from build123d import *

# Parameters (mm, degrees)
SKETCH1_W           = 270
SKETCH1_H           = 35
BOSS_EXTRUDE1_DEPTH = 10
SKETCH2_W           = 270
SKETCH2_H           = 26
BOSS_EXTRUDE2_DEPTH = 1
CUT_EXTRUDE1_REACH  = 141.821
SKETCH3_R           = 1.75
CUT_EXTRUDE3_REACH  = 141.896
SKETCH4_R           = 8
SKETCH5_R           = 10
CUT_EXTRUDE4_DEPTH  = 1.5
CUT_EXTRUDE5_START  = -1.5
SKETCH6_R           = 10
CUT_EXTRUDE5_DEPTH  = 1.5
CUT_EXTRUDE14_REACH = 141.896
SKETCH20_W          = 17
SKETCH20_H          = 15
BOSS_EXTRUDE5_DEPTH = 11
SKETCH21_R          = 4.25
CUT_EXTRUDE15_DEPTH = 9
FILLET1_R           = 7
CUT_EXTRUDE16_REACH = 146.381
SKETCH22_R          = 1.75
SKETCH24_R          = 3
CUT_EXTRUDE17_DEPTH = 5
BOSS_EXTRUDE6_DEPTH = 11
FILLET2_R           = 20
FILLET3_R           = 30
CHAMFER1_SIZE       = 1


# Some blends are built 0.0001 mm under size
with BuildPart() as part:
    # Sketch1 → Boss-Extrude1 (new body)
    with BuildSketch(Plane.XY):
        with Locations((0, -17.5)):
            Rectangle(SKETCH1_W, SKETCH1_H)
    extrude(amount=BOSS_EXTRUDE1_DEPTH)

    # Sketch2 → Boss-Extrude2 (add)
    with BuildSketch(Plane.XY.offset(10)):
        with Locations((0, -22)):
            Rectangle(SKETCH2_W, SKETCH2_H)
    extrude(amount=BOSS_EXTRUDE2_DEPTH)

    # Sketch3 → Cut-Extrude1 (cut, up to next)
    with BuildSketch(Plane.XY.offset(10), mode=Mode.PRIVATE) as cut_extrude1_sk1:
        with Locations((-130, -4.5)):
            Circle(SKETCH3_R)
    cut_extrude1_tool1 = extrude(cut_extrude1_sk1.sketch, amount=-CUT_EXTRUDE1_REACH, mode=Mode.PRIVATE) & part.part
    # Sketch3 → Cut-Extrude1 (cut, up to next)
    with BuildSketch(Plane.XY.offset(10), mode=Mode.PRIVATE) as cut_extrude1_sk2:
        with Locations((-110, -4.5)):
            Circle(SKETCH3_R)
    cut_extrude1_tool2 = extrude(cut_extrude1_sk2.sketch, amount=-CUT_EXTRUDE1_REACH, mode=Mode.PRIVATE) & part.part
    # Sketch3 → Cut-Extrude1 (cut, up to next)
    with BuildSketch(Plane.XY.offset(10), mode=Mode.PRIVATE) as cut_extrude1_sk3:
        with Locations((-90, -4.5)):
            Circle(SKETCH3_R)
    cut_extrude1_tool3 = extrude(cut_extrude1_sk3.sketch, amount=-CUT_EXTRUDE1_REACH, mode=Mode.PRIVATE) & part.part
    # Sketch3 → Cut-Extrude1 (cut, up to next)
    with BuildSketch(Plane.XY.offset(10), mode=Mode.PRIVATE) as cut_extrude1_sk4:
        with Locations((-70, -4.5)):
            Circle(SKETCH3_R)
    cut_extrude1_tool4 = extrude(cut_extrude1_sk4.sketch, amount=-CUT_EXTRUDE1_REACH, mode=Mode.PRIVATE) & part.part
    # Sketch3 → Cut-Extrude1 (cut, up to next)
    with BuildSketch(Plane.XY.offset(10), mode=Mode.PRIVATE) as cut_extrude1_sk5:
        with Locations((-50, -4.5)):
            Circle(SKETCH3_R)
    cut_extrude1_tool5 = extrude(cut_extrude1_sk5.sketch, amount=-CUT_EXTRUDE1_REACH, mode=Mode.PRIVATE) & part.part
    # Sketch3 → Cut-Extrude1 (cut, up to next)
    with BuildSketch(Plane.XY.offset(10), mode=Mode.PRIVATE) as cut_extrude1_sk6:
        with Locations((-30, -4.5)):
            Circle(SKETCH3_R)
    cut_extrude1_tool6 = extrude(cut_extrude1_sk6.sketch, amount=-CUT_EXTRUDE1_REACH, mode=Mode.PRIVATE) & part.part
    # Sketch3 → Cut-Extrude1 (cut, up to next)
    with BuildSketch(Plane.XY.offset(10), mode=Mode.PRIVATE) as cut_extrude1_sk7:
        with Locations((-10, -4.5)):
            Circle(SKETCH3_R)
    cut_extrude1_tool7 = extrude(cut_extrude1_sk7.sketch, amount=-CUT_EXTRUDE1_REACH, mode=Mode.PRIVATE) & part.part
    # Sketch3 → Cut-Extrude1 (cut, up to next)
    with BuildSketch(Plane.XY.offset(10), mode=Mode.PRIVATE) as cut_extrude1_sk8:
        with Locations((10, -4.5)):
            Circle(SKETCH3_R)
    cut_extrude1_tool8 = extrude(cut_extrude1_sk8.sketch, amount=-CUT_EXTRUDE1_REACH, mode=Mode.PRIVATE) & part.part
    # Sketch3 → Cut-Extrude1 (cut, up to next)
    with BuildSketch(Plane.XY.offset(10), mode=Mode.PRIVATE) as cut_extrude1_sk9:
        with Locations((30, -4.5)):
            Circle(SKETCH3_R)
    cut_extrude1_tool9 = extrude(cut_extrude1_sk9.sketch, amount=-CUT_EXTRUDE1_REACH, mode=Mode.PRIVATE) & part.part
    # Sketch3 → Cut-Extrude1 (cut, up to next)
    with BuildSketch(Plane.XY.offset(10), mode=Mode.PRIVATE) as cut_extrude1_sk10:
        with Locations((50, -4.5)):
            Circle(SKETCH3_R)
    cut_extrude1_tool10 = extrude(cut_extrude1_sk10.sketch, amount=-CUT_EXTRUDE1_REACH, mode=Mode.PRIVATE) & part.part
    # Sketch3 → Cut-Extrude1 (cut, up to next)
    with BuildSketch(Plane.XY.offset(10), mode=Mode.PRIVATE) as cut_extrude1_sk11:
        with Locations((70, -4.5)):
            Circle(SKETCH3_R)
    cut_extrude1_tool11 = extrude(cut_extrude1_sk11.sketch, amount=-CUT_EXTRUDE1_REACH, mode=Mode.PRIVATE) & part.part
    # Sketch3 → Cut-Extrude1 (cut, up to next)
    with BuildSketch(Plane.XY.offset(10), mode=Mode.PRIVATE) as cut_extrude1_sk12:
        with Locations((90, -4.5)):
            Circle(SKETCH3_R)
    cut_extrude1_tool12 = extrude(cut_extrude1_sk12.sketch, amount=-CUT_EXTRUDE1_REACH, mode=Mode.PRIVATE) & part.part
    add(cut_extrude1_tool1.solids().sort_by_distance((-130, -4.5, 10))[0], mode=Mode.SUBTRACT)
    add(cut_extrude1_tool2.solids().sort_by_distance((-110, -4.5, 10))[0], mode=Mode.SUBTRACT)
    add(cut_extrude1_tool3.solids().sort_by_distance((-90, -4.5, 10))[0], mode=Mode.SUBTRACT)
    add(cut_extrude1_tool4.solids().sort_by_distance((-70, -4.5, 10))[0], mode=Mode.SUBTRACT)
    add(cut_extrude1_tool5.solids().sort_by_distance((-50, -4.5, 10))[0], mode=Mode.SUBTRACT)
    add(cut_extrude1_tool6.solids().sort_by_distance((-30, -4.5, 10))[0], mode=Mode.SUBTRACT)
    add(cut_extrude1_tool7.solids().sort_by_distance((-10, -4.5, 10))[0], mode=Mode.SUBTRACT)
    add(cut_extrude1_tool8.solids().sort_by_distance((10, -4.5, 10))[0], mode=Mode.SUBTRACT)
    add(cut_extrude1_tool9.solids().sort_by_distance((30, -4.5, 10))[0], mode=Mode.SUBTRACT)
    add(cut_extrude1_tool10.solids().sort_by_distance((50, -4.5, 10))[0], mode=Mode.SUBTRACT)
    add(cut_extrude1_tool11.solids().sort_by_distance((70, -4.5, 10))[0], mode=Mode.SUBTRACT)
    add(cut_extrude1_tool12.solids().sort_by_distance((90, -4.5, 10))[0], mode=Mode.SUBTRACT)

    # Sketch4 → Cut-Extrude3 (cut, up to next)
    with BuildSketch(Plane.XY.offset(11), mode=Mode.PRIVATE) as cut_extrude3_sk1:
        with Locations((123, -24.5)):
            Circle(SKETCH4_R)
    cut_extrude3_tool1 = extrude(cut_extrude3_sk1.sketch, amount=-CUT_EXTRUDE3_REACH, mode=Mode.PRIVATE) & part.part
    add(cut_extrude3_tool1.solids().sort_by_distance((123, -24.5, 11))[0], mode=Mode.SUBTRACT)

    # Sketch5 → Cut-Extrude4 (cut)
    with BuildSketch(Plane.XY.offset(11)):
        with Locations((123, -24.5)):
            Circle(SKETCH5_R)
    extrude(amount=-CUT_EXTRUDE4_DEPTH, mode=Mode.SUBTRACT)

    # Sketch6 → Cut-Extrude5 (cut)
    with BuildSketch(Plane(origin=(0, 0, 0), x_dir=(-1, 0, 0), z_dir=(0, 0, -1)).offset(CUT_EXTRUDE5_START)):
        with Locations(Location((-123, -24.5, 0), (0, 0, 180))):
            Circle(SKETCH6_R)
    extrude(amount=CUT_EXTRUDE5_DEPTH, mode=Mode.SUBTRACT)

    # Sketch19 → Cut-Extrude14 (cut, up to next)
    with BuildSketch(Plane.XY.offset(11), mode=Mode.PRIVATE) as cut_extrude14_sk1:
        with BuildLine():
            Line((-135, -12), (-135, -35))
            Line((-135, -35), (-126.157637496, -35))
            ThreePointArc((-126.157637496, -35), (-129.258467146, -22.992390109), (-135, -12))
        make_face()
    cut_extrude14_tool1 = extrude(cut_extrude14_sk1.sketch, amount=-CUT_EXTRUDE14_REACH, mode=Mode.PRIVATE) & part.part
    add(cut_extrude14_tool1.solids().sort_by_distance((-131.679264, -26.580863, 11))[0], mode=Mode.SUBTRACT)

    # Sketch20 → Boss-Extrude5 (add)
    with BuildSketch(Plane.XY.offset(11)):
        with Locations((-89.087637496, -42.5)):
            Rectangle(SKETCH20_W, SKETCH20_H)
    extrude(amount=-BOSS_EXTRUDE5_DEPTH)

    # Sketch21 → Cut-Extrude15 (cut)
    with BuildSketch(Plane(origin=(0, 0, 0), x_dir=(-1, 0, 0), z_dir=(0, 0, -1))):
        with Locations((89.087637496, -41)):
            Circle(SKETCH21_R)
    extrude(amount=-CUT_EXTRUDE15_DEPTH, mode=Mode.SUBTRACT)

    # Fillet1
    fillet1_edges = [part.edges().sort_by_distance(p)[0] for p in [
        (-80.587637496, -50, 5.5),
        (-80.587637496, -35, 5.5),
        (-97.587637496, -35, 5.5),
        (-97.587637496, -50, 5.5),
    ]]
    fillet(fillet1_edges, radius=FILLET1_R)

    # Sketch22 → Cut-Extrude16 (cut, up to next)
    with BuildSketch(Plane.XY.offset(11), mode=Mode.PRIVATE) as cut_extrude16_sk1:
        with Locations((-75, -27)):
            Circle(SKETCH22_R)
    cut_extrude16_tool1 = extrude(cut_extrude16_sk1.sketch, amount=-CUT_EXTRUDE16_REACH, mode=Mode.PRIVATE) & part.part
    add(cut_extrude16_tool1.solids().sort_by_distance((-75, -27, 11))[0], mode=Mode.SUBTRACT)

    # Sketch24 → Cut-Extrude17 (cut)
    with BuildSketch(Plane.XY.offset(11)):
        with Locations((-75, -27)):
            Circle(SKETCH24_R)
    extrude(amount=-CUT_EXTRUDE17_DEPTH, mode=Mode.SUBTRACT)

    # Sketch25 → Boss-Extrude6 (add)
    with BuildSketch(Plane.XY.offset(11)):
        with BuildLine():
            Line((109.630258043, -35), (135, -35))
            Line((135, -35), (135, -12.458405421))
            ThreePointArc((135, -12.458405421), (134.291586239, -37.208268183), (109.630258043, -35))
        make_face()
    extrude(amount=-BOSS_EXTRUDE6_DEPTH)

    # Fillet2
    fillet2_edges = [part.edges().sort_by_distance(p)[0] for p in [
        (109.630258043, -35, 5.5),
        (135, -12.458405421, 5.5),
    ]]
    fillet(fillet2_edges, radius=FILLET2_R)

    # Fillet3
    # the kernel refuses this fillet: 30 mm, written as the material it takes off along each edge
    with BuildSketch(Plane(origin=(135, 0, -59.556893558), x_dir=(0.15687721441573954, -0.9876181142512312, 0), z_dir=(0, 0, 1))) as fillet3_piece_1:
        with BuildLine():
            CenterArc((25.891295603, -28.234103195), FILLET3_R, 109.756652653, 61.217662553)
            Line((-3.737247824, -23.527786763), (-6.700102167, -23.057155119))
            Line((-6.700102167, -23.057155119), (-2.962854343, 0.470631643))
            Line((-2.962854343, 0.470631643), (0.470631643, 2.962854343))
            ThreePointArc((0.470631643, 2.962854343), (6.323083142, 2.033227521), (14.736437724, 2.823410319))
            Line((14.736437724, 2.823410319), (15.750515713, 0))
        make_face()
    extrude(amount=129.113787116, mode=Mode.SUBTRACT)

    # Chamfer1
    chamfer1_edges = [part.edges().sort_by_distance(p)[0] for p in [
        (-97.587637496, -42.5, 11),
        (-89.087637496, -50, 11),
        (-80.587637496, -42.5, 11),
        (14.233001219, -35, 11),
        (-82.637890028, -47.949747468, 11),
        (-95.537384964, -47.949747468, 11),
        (-99.637890028, -37.050252532, 11),
        (-78.537384964, -37.050252532, 11),
        (-78, -27, 11),
        (-135, -10.5, 11),
        (134.556244982, -36.96808734, 11),
        (107.981129718, -35.898563801, 11),
        (137.585590708, -15.761389895, 11),
        (-1.199236069, -9, 11),
        (135.260308634, -12.111290452, 11),
        (113, -24.5, 11),
        (-115.372637496, -35, 11),
        (-129.258467146, -22.992390109, 11),
    ]]
    chamfer(chamfer1_edges, length=CHAMFER1_SIZE - 0.0001)  # a hair under: the kernel refuses the full size


solid = part.part
Could you check a few things on this model? Use its own coordinates, in mm. A direction names the side the tool comes from. Give positions to 0.01 mm unless a question says otherwise; leave off trailing zeros. Answer as CSV lines item,"result". Start each with the question number.
(1) If we mould it in two halves opening along Y, with no side actions, what happens to faces 1 (the face through (130.39, -27.56, 5.56)), 2 (the face through (4, -19, 0)), 3 (the face through (126.65, -4.3, 4.93))? For each: +Y half, -Y half, draft (parallel to the pull), parting line (faces both ways), or undercut.
(2) I'm going to push flat-ended pins straight in: pin 1 Ø10 at (x, y) = (120, -21) entering from -Z; pin 2 Ø5.5 at (x, y) = (-70, -4.5) entering from +Z; pin 3 Ø1 at (y, z) = (-20, 8.5) entering from -X. Where does each tip first touch, or does it pass through?
(3) Please list where these lines run through material, in increasing order: line 1 (Y direction, x = -50, z = 3.75); line 2 (X direction, y = -26, z = 5.5); line 3 (X direction, y = -10.5, z = 7).
(4) Which directions (+Z, -Z, +X, -X, +Y, -Y) give clear straight access to the entire face, cutting with the end or side of a thin tool? Please do faces 4 (the face through (-3, -4, 10)), 5 (the face through (-78.59, -36.88, 10.16)), 6 (the face through (13, -35, 5)).
Answer list:
1,face 1,"undercut"
1,face 2,"draft"
1,face 3,"+Y half"
2,pin 1,"z = 1.5"
2,pin 2,"z = 10"
2,pin 3,"x = -130.74"
3,line 1,"-35 to -6.25, -2.75 to 0"
3,line 2,"-128.2 to -76.44, -73.56 to 115.14, 130.86 to 139.93"
3,line 3,"-135 to 133.98"
4,face 4,"+Z, +X, -X, +Y"
4,face 5,"+Z, -Y"
4,face 6,"+Z, -Z, -Y"
